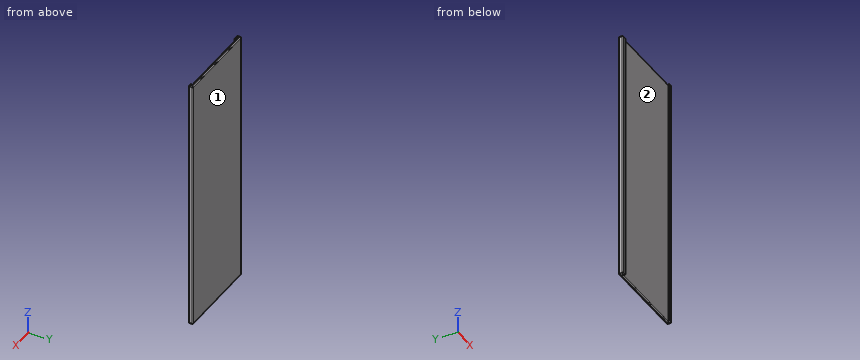
from build123d import *

# Parameters (mm, degrees)
F1_DEPTH = 150
F2_R     = 0.5


with BuildPart() as f1:
    # F0 (on Top) → F1 (new body)
    with BuildSketch(Plane.XY):
        Polygon((1, -1), (0, 0), (47, 0), (46, -1), (48.5, -1), (48.5, 1.5), (-1.5, 1.5), (-1.5, -1), align=None)
    extrude(amount=F1_DEPTH)

    # F2
    f2_edges = [f1.edges().sort_by_distance(p)[0] for p in [
        (23.5, 0, 150),
        (23.5, 1.5, 150),
        (-1.5, 0.25, 150),
        (48.5, 0.25, 150),
        (48.5, -1, 75),
        (48.5, 1.5, 75),
        (48.5, 0.25, 0),
        (-1.5, -1, 75),
        (-1.5, 1.5, 75),
        (23.5, 1.5, 0),
        (-1.5, 0.25, 0),
        (47.25, -1, 0),
        (-0.25, -1, 0),
        (23.5, 0, 0),
        (-0.25, -1, 150),
        (47.25, -1, 150),
    ]]
    fillet(f2_edges, radius=F2_R)


solid = f1.part
Source: CAD feature listing. Evaluate the final solid. Frame: model axes, mm. Face numbers are marked on the shaded views. Give positions to 0.01 mm unless a question says otherwise; leave off trailing zeros. Write each loop counter-clockwise with the first axis right and the second up, starting at its lowest first coordinate (ties: lowest second). Pieces come first, ordered by that corner, then holes. Notation, with made-up numbers: (-11.5, -4.75) -> (4.5, -4.75) arc R8 cw to (4.5, 7.25) -> close; hole circle Ø1 at (55, 63.25). An arc over 180 degrees is marked (long way). Return JSON: item names as keys, results as strings. Group by question number.
1. Material intervals for line 1 (Y direction, x = 35.5, z = 30); line 2 (X direction, y = -0.35, z = 94); line 3 (X direction, y = 1.15, z = 66), sorted ascending. Write a range as from..to.
2. Mould query, pull axis X, two halves, no side actions, for the marked faces 1 and 2. Classes: +X half, -X half, draft (parallel to the pull), parting line (faces both ways), or undercut.
3. Pin query (flat end, axial travel): pin 1 Ø1 at (x, z) = (12, 16.5) entering from -Y. Return the tip coordinate at first contact, or that it passes through.
4. Section B-B, the plane z = 70. Output: boundary loops of the cut face in (x, y), then the cut area to 3 significant figures.
5. Section A-A, the plane x = 34. Output: boundary loops of the cut face in (y, z).
Determined:
{
 "1": {"line 1": "y = 0..1.5", "line 2": "x = -1.5..0.35, 46.65..48.5", "line 3": "x = -1.48..48.48"},
 "2": {"face 1": "draft", "face 2": "undercut"},
 "3": {"pin 1": "stops at y = 0"},
 "4": {"outline": "(-1.5, -0.5) arc R0.5 ccw to (-1, -1) -> (1, -1) -> (0, 0) -> (47, 0) -> (46, -1) -> (48, -1) arc R0.5 ccw to (48.5, -0.5) -> (48.5, 1) arc R0.5 ccw to (48, 1.5) -> (-1, 1.5) arc R0.5 ccw to (-1.5, 1) -> close", "area": "78.8 mm2"},
 "5": {"outline": "(0, 0.5) arc R0.5 ccw to (0.5, 0) -> (1, 0) arc R0.5 ccw to (1.5, 0.5) -> (1.5, 149.5) arc R0.5 ccw to (1, 150) -> (0.5, 150) arc R0.5 ccw to (0, 149.5) -> close"}
}
